Geometry: final body of the model. Coordinates: model frame, mm. A direction names the side the tool comes from. Coordinates: 2 decimals unless noted, no trailing zeros. Write each loop counter-clockwise with the first axis right and the second up, starting at its lowest first coordinate (ties: lowest second). Pieces come first, ordered by that corner, then holes. Notation, with made-up numbers: (-26, 33.25) - (23, 33.25) arc R25 cw to (23, 47.25) - close; hole circle Ø7 at (42.5, 81.5). An arc over 180 degrees is marked (long way). Put each result on its own line as item: value.
```python
from build123d import *

# Parameters (mm, degrees)
SKIZZE1_W                       = 20.3
SKIZZE1_H                       = 20.3
AUFSATZ_LINEAR_AUSTRAGEN1_DEPTH = 10
VERRUNDUNG1_R                   = 0.2
VERRUNDUNG2_R                   = 2.5
SKIZZE2_R                       = 2.3
SCHNITT_LINEAR_AUSTRAGEN1_DEPTH = 58.614695391
SKETCH1_R                       = 3.75
CUT_EXTRUDE1_DEPTH              = 8.025
CUT_EXTRUDE2_START              = -42.725
SKETCH1_2_R                     = 3.75
CUT_EXTRUDE2_DEPTH              = 8.025
FASE2_SIZE                      = 0.5


with BuildPart() as part:
    # Skizze1 → Aufsatz-Linear austragen1 (new body)
    with BuildSketch(Plane.XY):
        with BuildLine():
            Line((17.807565106, 25.375), (-17.807565106, 25.375))
            ThreePointArc((-17.807565106, 25.375), (-21.920310217, 21.920310217), (-25.375, 17.807565106))
            Line((-25.375, 17.807565106), (-25.375, -17.807565106))
            ThreePointArc((-25.375, -17.807565106), (-21.920310217, -21.920310217), (-17.807565106, -25.375))
            Line((-17.807565106, -25.375), (17.807565106, -25.375))
            ThreePointArc((17.807565106, -25.375), (21.920310217, -21.920310217), (25.375, -17.807565106))
            Line((25.375, -17.807565106), (25.375, 17.807565106))
            ThreePointArc((25.375, 17.807565106), (21.920310217, 21.920310217), (17.807565106, 25.375))
        make_face()
        Rectangle(SKIZZE1_W, SKIZZE1_H, mode=Mode.SUBTRACT)
    extrude(amount=AUFSATZ_LINEAR_AUSTRAGEN1_DEPTH)

    # Verrundung1
    verrundung1_edges = [part.edges().sort_by_distance(p)[0] for p in [
        (10.15, -10.15, 5),
        (10.15, 10.15, 5),
        (-10.15, 10.15, 5),
        (-10.15, -10.15, 5),
    ]]
    fillet(verrundung1_edges, radius=VERRUNDUNG1_R)

    # Verrundung2
    verrundung2_edges = [part.edges().sort_by_distance(p)[0] for p in [
        (25.375, 17.807565106, 5),
        (25.375, -17.807565106, 5),
        (17.807565106, -25.375, 5),
        (-17.807565106, -25.375, 5),
        (-25.375, -17.807565106, 5),
        (-25.375, 17.807565106, 5),
        (-17.807565106, 25.375, 5),
        (17.807565106, 25.375, 5),
    ]]
    fillet(verrundung2_edges, radius=VERRUNDUNG2_R)

    # Skizze2 → Schnitt-Linear austragen1 (cut, through all)
    with BuildSketch(Plane(origin=(25.375, 0, 0), x_dir=(0, 0, -1), z_dir=(1, 0, 0))):
        with Locations(Location((-5, 0, 0), (0, 0, 90))):
            Circle(SKIZZE2_R)
    extrude(amount=-SCHNITT_LINEAR_AUSTRAGEN1_DEPTH, mode=Mode.SUBTRACT)

    # Sketch1 → Cut-Extrude1 (cut)
    with BuildSketch(Plane.ZY.offset(25.375)):
        with Locations((5, 0)):
            Circle(SKETCH1_R)
    extrude(amount=-CUT_EXTRUDE1_DEPTH, mode=Mode.SUBTRACT)

    # Sketch1<2> → Cut-Extrude2 (cut)
    with BuildSketch(Plane.ZY.offset(25.375).offset(CUT_EXTRUDE2_START)):
        with Locations((5, 0)):
            Circle(SKETCH1_2_R)
    extrude(amount=-CUT_EXTRUDE2_DEPTH, mode=Mode.SUBTRACT)

    # Fase2
    fase2_edges = [part.edges().sort_by_distance(p)[0] for p in [
        (-10.15, -2.3, 5),
        (10.15, -2.3, 5),
        (-17.35, -2.3, 5),
        (17.35, -2.3, 5),
        (0, -10.15, 0),
        (0, -10.15, 10),
        (10.15, 0, 0),
        (10.15, 0, 10),
        (-10.15, 0, 0),
        (-10.15, 0, 10),
        (0, 10.15, 0),
        (0, 10.15, 10),
        (10.091421356, -10.091421356, 0),
        (10.091421356, -10.091421356, 10),
        (-10.091421356, -10.091421356, 0),
        (-10.091421356, -10.091421356, 10),
        (-10.091421356, 10.091421356, 0),
        (-10.091421356, 10.091421356, 10),
        (10.091421356, 10.091421356, 0),
        (10.091421356, 10.091421356, 10),
        (0, 25.375, 0),
        (0, 25.375, 10),
        (21.920310217, 21.920310217, 0),
        (25.375, 0, 0),
        (21.920310217, -21.920310217, 0),
        (0, -25.375, 0),
        (-21.920310217, -21.920310217, 0),
        (-25.375, 0, 0),
        (-21.920310217, 21.920310217, 0),
        (-17.784891513, 25.248441317, 0),
        (-25.248441317, 17.784891513, 0),
        (-25.248441317, -17.784891513, 0),
        (-17.784891513, -25.248441317, 0),
        (17.784891513, -25.248441317, 0),
        (25.248441317, -17.784891513, 0),
        (25.248441317, 17.784891513, 0),
        (17.784891513, 25.248441317, 0),
        (21.920310217, 21.920310217, 10),
        (-21.920310217, 21.920310217, 10),
        (-25.375, 0, 10),
        (-21.920310217, -21.920310217, 10),
        (0, -25.375, 10),
        (21.920310217, -21.920310217, 10),
        (25.375, 0, 10),
        (-17.784891513, 25.248441317, 10),
        (-25.248441317, 17.784891513, 10),
        (-25.248441317, -17.784891513, 10),
        (-17.784891513, -25.248441317, 10),
        (17.784891513, -25.248441317, 10),
        (25.248441317, -17.784891513, 10),
        (25.248441317, 17.784891513, 10),
        (17.784891513, 25.248441317, 10),
    ]]
    chamfer(fase2_edges, length=FASE2_SIZE)


solid = part.part
```
1. Ray query, probe 1 along Y at (x, z) = (-6.5, 2.75) (3 decimals); probe 2 along Z at (x, y) = (12.5, 0). Return the intervals inside material, ascending. Write a range as from..to.
Answer below:
probe 1: y = -25.375..-10.15, 10.15..25.375
probe 2: z = 0..2.7, 7.3..10
2. Section query A-A (x = 0). Return loops of the section in (y, z) (3 decimals).
Answer below:
outline: (-25.375, 0.5) - (-24.875, 0) - (-10.65, 0) - (-10.15, 0.5) - (-10.15, 9.5) - (-10.65, 10) - (-24.875, 10) - (-25.375, 9.5) - close; (10.15, 0.5) - (10.65, 0) - (24.875, 0) - (25.375, 0.5) - (25.375, 9.5) - (24.875, 10) - (10.65, 10) - (10.15, 9.5) - close
3. Section query C-C (y = 0). Count the separate pieces of the cut face and the enclosed holes in it, then the cut area to 3 significant figures.
Answer below:
separate pieces: 4
enclosed holes: 0
area: 116 mm²
4. Mould query, pull axis X, two halves, no side actions, for faces 1 (the cylindrical face through (-21.965, -21.875, 4.937)), 2 (the flat face through (-11, 0, 10)), 3 (the flat face through (0, -10.15, 5)). Classes: +X half, -X half, draft (parallel to the pull), parting line (faces both ways), or undercut.
Answer below:
face 1: -X half
face 2: draft
face 3: undercut
5. Pin query (flat end, axial travel): pin 1 Ø6 at (y, z) = (0, 5) entering from +X; pin 2 Ø2.5 at (y, z) = (-0.5, 6.5) entering from -X. Return the tip coordinate at first contact, or that it passes through.
Answer below:
pin 1: stops at x = 17.35
pin 2: stops at x = -17.35
6. Set-up query: faces 4 (the cylindrical face through (21.965, 21.875, 4.937)), 5 (the flat face through (17.35, 0, 2)), 6 (the flat face through (-17.35, 0, 2)). Return all of +Z, -Z, +X, -X, +Y, -Y with unobstructed straight access to the full face (end or side cutting, diameter ignored); none if empty.
Answer below:
face 4: +Z, -Z, +X, +Y
face 5: +X
face 6: -X
